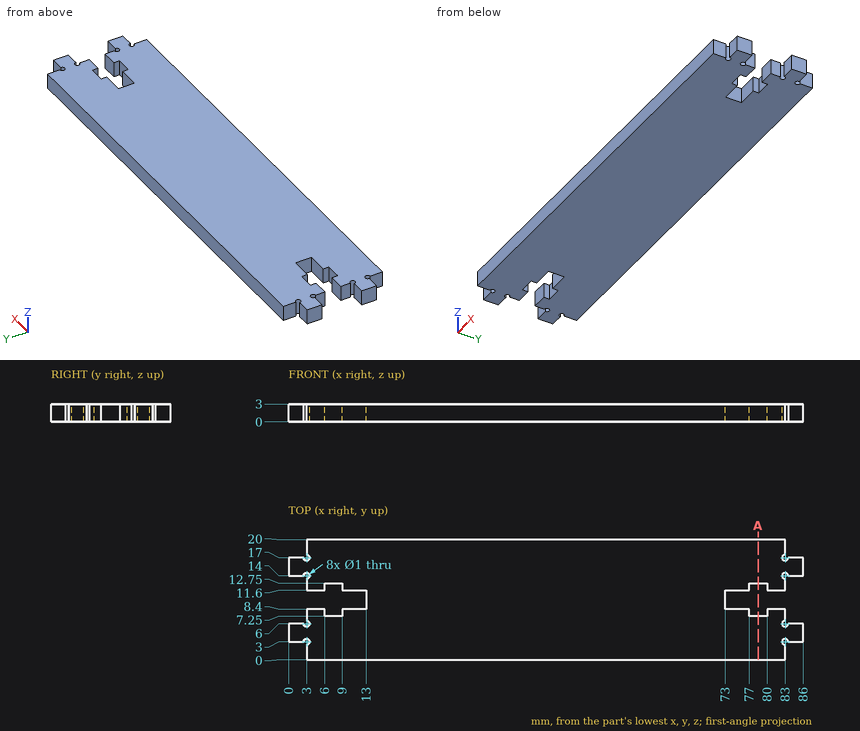
Design review of the part shown in the three views and the two pictorial views. Dimensions are in mm from the part's minimum x, y and z. Give positions to 0.01 mm unless a question says otherwise; leave off trailing zeros. Write each loop counter-clockwise with the first axis right and the second up, starting at its lowest first coordinate (ties: lowest second). Pieces come first, ordered by that corner, then holes.
(1) Add section A-A (x = 78.5). Give the boundary of the cut face in (y, z).
Checked values:
outline: (0, 0) - (7.25, 0) - (7.25, 3) - (0, 3) - close; (12.75, 0) - (20, 0) - (20, 3) - (12.75, 3) - close
(2) Wall thickness on line 1 along X through (y, z) = (12, 1.25); line 2 along Y through (x, z) = (77.5, 2.75); line 3 along Y through (x, z) = (5, 0.7): over which ranges is each line inside the solid? List them lowest first.
Checked values:
line 1: x = 3 to 6, 9 to 77, 80 to 83
line 2: y = 0 to 7.25, 12.75 to 20
line 3: y = 0 to 8.4, 11.6 to 20
(3) Clearance check with flat-ended pins moving along their axes: pin 1 Ø1.2 at (x, z) = (85.5, 1) entering from +Y; pin 2 Ø0.8 at (x, z) = (84.5, 2) entering from -Y; pin 3 Ø0.8 at (y, z) = (1.5, 2) entering from -X. State where each tip first meets the part, or that it passes through.
Checked values:
pin 1: stops at y = 17
pin 2: stops at y = 3
pin 3: stops at x = 3
